```python
from build123d import *

# Parameters (mm, degrees)
F0_W     = 50
F0_H     = 320
F1_DEPTH = 30
F2_W     = 20
F2_H     = 320
F3_DEPTH = 15
F4_R     = 9
F5_DEPTH = 30.001


with BuildPart() as f1:
    # F0 (on Top) → F1 (new body)
    with BuildSketch(Plane.XY):
        with Locations((25, 160)):
            Rectangle(F0_W, F0_H)
    extrude(amount=F1_DEPTH)

    # F2 (on face) → F3 (cut)
    with BuildSketch(Plane(origin=(0, 0, 0), x_dir=(1, 0, 0), z_dir=(0, 0, -1))):
        with Locations((25, -160)):
            Rectangle(F2_W, F2_H)
    extrude(amount=-F3_DEPTH, mode=Mode.SUBTRACT)

    # F4 (on face) → F5 (cut, through all)
    with BuildSketch(Plane.XY.offset(30)):
        with Locations((25, 50)):
            Circle(F4_R)
        with Locations((25, 90)):
            Circle(F4_R)
        with Locations((25, 130)):
            Circle(F4_R)
        with Locations((25, 170)):
            Circle(F4_R)
        with Locations((25, 210)):
            Circle(F4_R)
        with Locations((25, 250)):
            Circle(F4_R)
        with Locations((25, 290)):
            Circle(F4_R)
    extrude(amount=-F5_DEPTH, mode=Mode.SUBTRACT)


solid = f1.part
```
For this review, take the finished solid that the model builds, in its own axes (mm). A direction names the side the tool comes from. Round coordinates to 2 decimals unless told otherwise and drop trailing zeros. Write each loop counter-clockwise with the first axis right and the second up, starting at its lowest first coordinate (ties: lowest second). Pieces come first, ordered by that corner, then holes. Notation, with made-up numbers: M 13,-21.5 L 62,-21.5 A30 cw 62,8.5 Z; hole C -25.75,68.25 d1. An arc over 180 degrees is marked long. One line per item, written item: value. Start each with the question number.
(1) We need section D-D (y = 127). Give the boundary of the cut face in (x, z), and give its area (3 significant figures).
(2) We need section A-A (x = 25). Count the separate pieces of the cut face and the enclosed holes in it, and give its area (3 significant figures).
(3) Machinability: for faces 4 (the flat face through (15, 162, 7)), 5 (the cylindrical face through (29.84, 57.59, 22.6)), which of the approach directions +Z, -Z, +X, -X, +Y, -Y give a long, thin tool a straight path to every point of the face, cutting with its end or side? Answer none if there is none.
(4) Wall thickness on line 1 (X direction, y = 228.5, z = 3); line 2 (Z direction, x = 22.5, y = 268.5); line 3 (X direction, y = 163, z = 16): over which ranges is each line inside the solid? List them lowest first.
(5) Insertion check: pin 1 (8 mm diameter, centred on x = 24.5, y = 230.5, fed in from -Z). The pin has a flat end and moves straight along its axis. Give the tip position at first contact, or say it passes through.
(6) We need section C-C (z = 18). Give the boundary of the cut face in (x, y), and give its area (3 significant figures).
(7) The part is to be moulded in two halves that separate along Y. For faces 1 (the flat face through (25, 0, 18)), 2 (the flat face through (25, 193, 15)), 3 (the cylindrical face through (23.828, 218.923, 22.605)), say which applies: released by +Y, released by -Y, zero draft, split by the parting line, or undercut.
(8) We need section B-B (y = 50). Give the boundary of the cut face in (x, z), and give its area (3 significant figures).
Result:
1. outline: M 0,0 L 15,0 L 15,15 L 16.51,15 L 16.51,30 L 0,30 Z; M 33.49,15 L 35,15 L 35,0 L 50,0 L 50,30 L 33.49,30 Z
1. area: 945 mm²
2. separate pieces: 8
2. enclosed holes: 0
2. area: 2,910 mm²
3. face 4: -Z, +Y, -Y
3. face 5: +Z, -Z
4. line 1: 0 to 15, 35 to 50
4. line 2: 15 to 30
4. line 3: 0 to 19.34, 30.66 to 50
5. pin 1: z = 15
6. outline: M 0,0 L 50,0 L 50,320 L 0,320 Z; hole C 25,50 d18; hole C 25,90 d18; hole C 25,130 d18; hole C 25,170 d18; hole C 25,210 d18; hole C 25,250 d18; hole C 25,290 d18
6. area: 14,200 mm²
7. face 1: released by -Y
7. face 2: zero draft
7. face 3: undercut
8. outline: M 0,0 L 15,0 L 15,15 L 16,15 L 16,30 L 0,30 Z; M 34,15 L 35,15 L 35,0 L 50,0 L 50,30 L 34,30 Z
8. area: 930 mm²
